Part model, mm, in its own coordinate system. Face numbers are marked on the shaded views. A direction names the side the tool comes from. Give positions to 0.01 mm unless a question says otherwise; leave off trailing zeros. Write each loop counter-clockwise with the first axis right and the second up, starting at its lowest first coordinate (ties: lowest second). Pieces come first, ordered by that corner, then holes. Notation, with made-up numbers: (7.5, -36.75) - (60.5, -36.75) arc R11 ccw to (60.5, -20.75) - close; hole circle Ø5 at (-32.5, 12.5). An arc over 180 degrees is marked (long way). Answer as a JSON object with one key per item and string values. Group by question number.
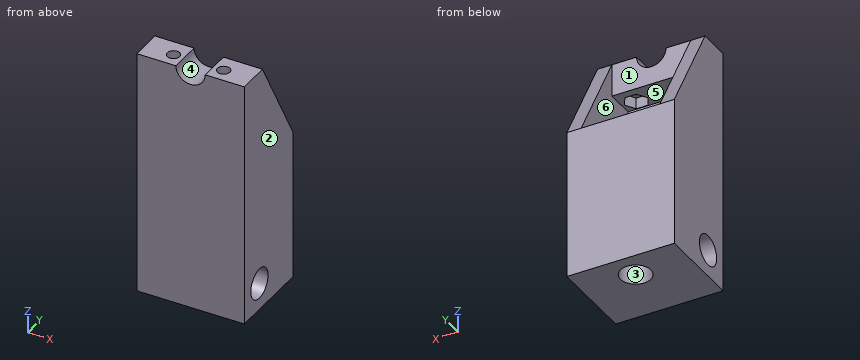
```python
from build123d import *

# Parameters (mm, degrees)
SCHIZZO7_W                   = 30
SCHIZZO7_H                   = 24.2
SCHIZZO7_R                   = 4.25
ESTRUSIONE_ESTRUSIONE3_DEPTH = 7.5
TAGLIO_ESTRUSIONE1_REACH     = 35.206
SCHIZZO8_R                   = 4.25
SCHIZZO12_W                  = 30
SCHIZZO12_H                  = 9
ESTRUSIONE_ESTRUSIONE5_DEPTH = 53.9
TAGLIO_ESTRUSIONE3_REACH     = 67.008
SCHIZZO15_W                  = 22
SCHIZZO15_H                  = 18
TAGLIO_ESTRUSIONE4_DEPTH     = 8
TAGLIO_ESTRUSIONE5_REACH     = 73.545
SCHIZZO16_R                  = 1.75
TAGLIO_ESTRUSIONE6_DEPTH     = 3.1
SCHIZZO20_W                  = 30
SCHIZZO20_H                  = 15.2
SCHIZZO20_R                  = 4.25
ESTRUSIONE_ESTRUSIONE6_DEPTH = 26.8
ESTRUSIONE_ESTRUSIONE7_DEPTH = 4
ESTRUSIONE_ESTRUSIONE8_START = -4
ESTRUSIONE_ESTRUSIONE8_DEPTH = 4


with BuildPart() as part:
    # Schizzo7 → Estrusione-Estrusione3 (new, symmetric)
    with BuildSketch(Plane.XY):
        Rectangle(SCHIZZO7_W, SCHIZZO7_H)
        with Locations((0, 4.6)):
            Circle(SCHIZZO7_R, mode=Mode.SUBTRACT)
    extrude(amount=ESTRUSIONE_ESTRUSIONE3_DEPTH, both=True)

    # Schizzo8 → Taglio-Estrusione1 (cut, up to next)
    with BuildSketch(Plane(origin=(15, 0, 0), x_dir=(0, 0, -1), z_dir=(1, 0, 0)), mode=Mode.PRIVATE) as taglio_estrusione1_sk1:
        with Locations((0, -4.6)):
            Circle(SCHIZZO8_R)
    taglio_estrusione1_tool1 = extrude(taglio_estrusione1_sk1.sketch, amount=-TAGLIO_ESTRUSIONE1_REACH, mode=Mode.PRIVATE) & part.part
    add(taglio_estrusione1_tool1.solids().sort_by_distance((15, -4.6, 0))[0], mode=Mode.SUBTRACT)

    # Schizzo12 → Estrusione-Estrusione5 (add)
    with BuildSketch(Plane.XY.offset(7.5)):
        with Locations((0, -7.6)):
            Rectangle(SCHIZZO12_W, SCHIZZO12_H)
    extrude(amount=ESTRUSIONE_ESTRUSIONE5_DEPTH)

    # Schizzo14 → Taglio-Estrusione3 (cut, up to next)
    with BuildSketch(Plane(origin=(0, -3.1, 0), x_dir=(1, 0, 0), z_dir=(0, 1, 0)), mode=Mode.PRIVATE) as taglio_estrusione3_sk1:
        with BuildLine():
            Line((4.1, -61.4), (-4.1, -61.4))
            ThreePointArc((-4.1, -61.4), (0, -57.3), (4.1, -61.4))
        make_face()
    taglio_estrusione3_tool1 = extrude(taglio_estrusione3_sk1.sketch, amount=-TAGLIO_ESTRUSIONE3_REACH, mode=Mode.PRIVATE) & part.part
    add(taglio_estrusione3_tool1.solids().sort_by_distance((0, -3.1, 59.659906))[0], mode=Mode.SUBTRACT)

    # Schizzo15 → Taglio-Estrusione4 (cut)
    with BuildSketch(Plane(origin=(0, -3.1, 0), x_dir=(1, 0, 0), z_dir=(0, 1, 0))):
        with Locations((0, -43.3)):
            Rectangle(SCHIZZO15_W, SCHIZZO15_H)
    extrude(amount=-TAGLIO_ESTRUSIONE4_DEPTH, mode=Mode.SUBTRACT)

    # Schizzo16 → Taglio-Estrusione5 (cut, up to next)
    with BuildSketch(Plane.XY.offset(61.4), mode=Mode.PRIVATE) as taglio_estrusione5_sk1:
        with Locations((-7, -8.1)):
            Circle(SCHIZZO16_R)
    taglio_estrusione5_tool1 = extrude(taglio_estrusione5_sk1.sketch, amount=-TAGLIO_ESTRUSIONE5_REACH, mode=Mode.PRIVATE) & part.part
    # Schizzo16 → Taglio-Estrusione5 (cut, up to next)
    with BuildSketch(Plane.XY.offset(61.4), mode=Mode.PRIVATE) as taglio_estrusione5_sk2:
        with Locations((7, -8.1)):
            Circle(SCHIZZO16_R)
    taglio_estrusione5_tool2 = extrude(taglio_estrusione5_sk2.sketch, amount=-TAGLIO_ESTRUSIONE5_REACH, mode=Mode.PRIVATE) & part.part
    add(taglio_estrusione5_tool1.solids().sort_by_distance((-7, -8.1, 61.4))[0], mode=Mode.SUBTRACT)
    add(taglio_estrusione5_tool2.solids().sort_by_distance((7, -8.1, 61.4))[0], mode=Mode.SUBTRACT)

    # Schizzo17 → Taglio-Estrusione6 (cut)
    with BuildSketch(Plane(origin=(0, 0, 52.3), x_dir=(-1, 0, 0), z_dir=(0, 0, -1))):
        Polygon((-3.75, -8.1), (-5.375, -5.285417438), (-8.625, -5.285417438), (-10.25, -8.1), (-8.625, -10.914582562), (-5.375, -10.914582562), align=None)
        Polygon((5.375, -10.914582562), (3.75, -8.1), (5.375, -5.285417438), (8.625, -5.285417438), (10.25, -8.1), (8.625, -10.914582562), align=None)
    extrude(amount=-TAGLIO_ESTRUSIONE6_DEPTH, mode=Mode.SUBTRACT)

    # Schizzo20 → Estrusione-Estrusione6 (add)
    with BuildSketch(Plane.XY.offset(7.5)):
        with Locations((0, 4.5)):
            Rectangle(SCHIZZO20_W, SCHIZZO20_H)
        with Locations((0, 4.6)):
            Circle(SCHIZZO20_R, mode=Mode.SUBTRACT)
    extrude(amount=ESTRUSIONE_ESTRUSIONE6_DEPTH)

    # Schizzo21 → Estrusione-Estrusione7 (add)
    with BuildSketch(Plane.ZY.offset(15)):
        Polygon((34.3, 12.1), (61.4, -3.1), (34.3, -3.1), align=None)
    extrude(amount=-ESTRUSIONE_ESTRUSIONE7_DEPTH)

    # Schizzo22 → Estrusione-Estrusione8 (add)
    with BuildSketch(Plane(origin=(15, 0, 0), x_dir=(0, 0, -1), z_dir=(1, 0, 0)).offset(ESTRUSIONE_ESTRUSIONE8_START)):
        Polygon((-34.3, 12.1), (-61.4, -3.1), (-34.3, -3.1), align=None)
    extrude(amount=ESTRUSIONE_ESTRUSIONE8_DEPTH)


solid = part.part
```
1) Which spindle directions (+Z, -Z, +X, -X, +Y, -Y) get a long thin tool onto all of the face, cutting with end or side? Do the marked faces 1 and 2. Say none if no direction does.
2) Drop flat-ended pins along their axis: P1, Ø13.5, axis at y = -4.6, z = 0, coming from the -X side; P2, Ø1, axis at x = 4.5, y = 8, coming from the +Z side; P3, Ø3.5, axis at x = 7.5, z = 54.5, coming from the +Y side; P4, Ø7.5, axis at x = 0, y = 4.6, coming from the +Z side. Give the stop position or say it passes through.
3) Saw through at B-B (z = 25.5). List the corners of the cut face in (x, y), and give its area (3 significant figures).
4) Two-plate mould, pull along Z, no slides. Class the marked faces 3, 4, 5 and 6: +Z half, -Z half, draft (parallel to the pull), parting line (faces both ways), or undercut.
5) Saw through at C-C (x = 0). List the corners of the cut face in (y, z).
6) Saw through at D-D (y = 1). List the corners of the cut face in (x, z), and give its area (3 significant figures).
7) Saw through at A-A (x = -7). List the corners of the cut face in (y, z).
8) Drill centre lines: line 1 along X through (y, z) = (-9, 39); line 2 along Y through (x, z) = (-7, 59.6); line 3 along Y through (x, z) = (0, 15.5). Where is each one in solid material? Low to high. Write a range as from..to.
Checks:
{
 "1": {"face 1": "+Z, +Y", "face 2": "+Z, -Z, +X, +Y, -Y"},
 "2": {"P1": "x = -15", "P2": "z = 34.3", "P3": "y = -3.1", "P4": "through"},
 "3": {"outline": "(-15, -12.1) - (15, -12.1) - (15, 12.1) - (-15, 12.1) - close; hole circle Ø8.5 at (0, 4.6)", "area": "669 mm2"},
 "4": {"face 3": "draft", "face 4": "+Z half", "face 5": "undercut", "face 6": "undercut"},
 "5": {"outline": "(-12.1, -7.5) - (0.35, -7.5) - (0.35, 34.3) - (-11.1, 34.3) - (-11.1, 52.3) - (-3.1, 52.3) - (-3.1, 57.3) - (-12.1, 57.3) - close; (8.85, -7.5) - (12.1, -7.5) - (12.1, 34.3) - (8.85, 34.3) - close; hole circle Ø8.5 at (-4.6, 0)"},
 "6": {"outline": "(-15, -7.5) - (-2.26, -7.5) - (-2.26, 34.3) - (-11, 34.3) - (-11, 54.09) - (-15, 54.09) - close; (2.26, -7.5) - (15, -7.5) - (15, 54.09) - (11, 54.09) - (11, 34.3) - (2.26, 34.3) - close", "area": "1,220 mm2"},
 "7": {"outline": "(-12.1, -7.5) - (12.1, -7.5) - (12.1, 34.3) - (-11.1, 34.3) - (-11.1, 52.3) - (-10.91, 52.3) - (-10.91, 55.4) - (-9.85, 55.4) - (-9.85, 61.4) - (-12.1, 61.4) - close; (-6.35, 55.4) - (-5.29, 55.4) - (-5.29, 52.3) - (-3.1, 52.3) - (-3.1, 61.4) - (-6.35, 61.4) - close; hole circle Ø8.5 at (-4.6, 0)"},
 "8": {"line 1": "-15..-11, 11..15", "line 2": "-12.1..-9.85, -6.35..-3.1", "line 3": "-12.1..0.35, 8.85..12.1"}
}
